Verification items for this drawing (mm, ordinates from the low corner). Give positions to 0.01 mm unless a question says otherwise; leave off trailing zeros. Write each loop counter-clockwise with the first axis right and the second up, starting at its lowest first coordinate (ties: lowest second). Pieces come first, ordered by that corner, then holes. Notation, with made-up numbers: M 58,55 L 96,55 A8 cw 96,60 Z; hole C 32.25,45.5 d3. An arc over 180 degrees is marked long. Write each question's results on one line, items separated by ' | '.
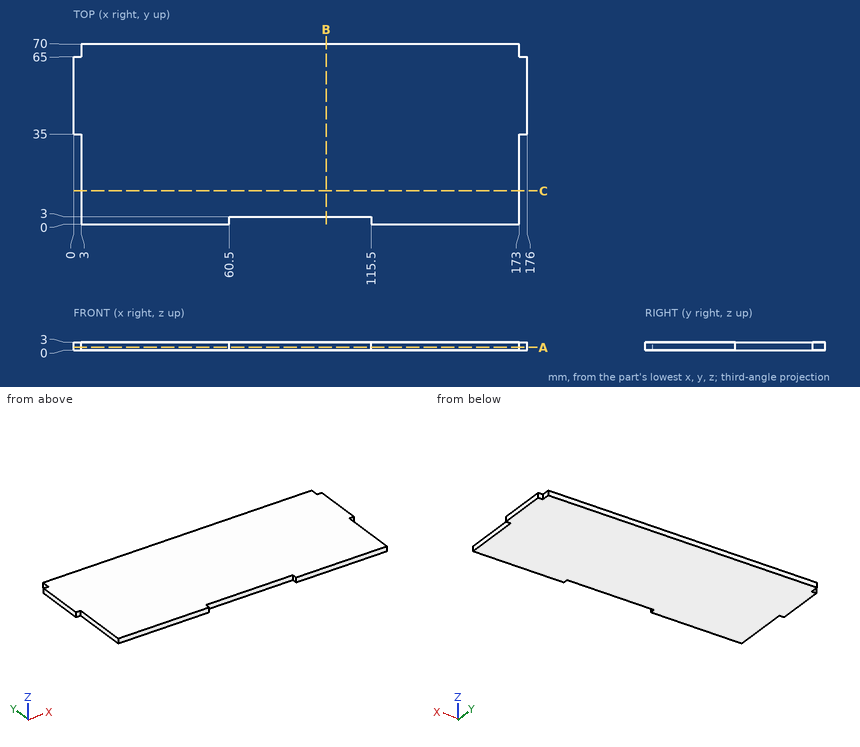
Q1. Depth check by flat-ended pin: P1, Ø1.5, axis at x = 88.5, z = 2, coming from the -Y side; P2, Ø1.5, axis at x = 1, z = 1.5, coming from the +Y side. Enter the tip coordinate at first touch or a pass-through.
Answer key:
P1: stops at y = 3 | P2: stops at y = 65
Q2. Section check A-A (z = 1.1). Enter the section's corners in (x, y).
Answer key:
outline: M 0,35 L 3,35 L 3,0 L 60.5,0 L 60.5,3 L 115.5,3 L 115.5,0 L 173,0 L 173,35 L 176,35 L 176,65 L 173,65 L 173,70 L 3,70 L 3,65 L 0,65 Z
Q3. Section check B-B (x = 98). Enter the section's corners in (y, z).
Answer key:
outline: M 3,0 L 70,0 L 70,3 L 3,3 Z
Q4. Material ranges on probe 1 along Y at (x, z) = (95, 1.8); probe 2 along X at (y, z) = (16.5, 0.4), recorded low to high. Write a range as [from, to].
Answer key:
probe 1: y = [3, 70] | probe 2: x = [3, 173]
Q5. Section check C-C (y = 13). Enter the section's corners in (x, z).
Answer key:
outline: M 3,0 L 173,0 L 173,3 L 3,3 Z
